from build123d import *

# Parameters (mm, degrees)
F1_DEPTH = 4
F2_R     = 5.08
F3_R     = 5.08
F4_R     = 1
F5_R     = 1
F6_R     = 1.5
F7_DEPTH = 25.4
F8_R     = 1


# Not quite as in the source:
# - a feature names something its author has since deleted; it is built from what else it names


with BuildPart() as f1:
    # F0 (on Top) → F1 (new body)
    with BuildSketch(Plane.XY):
        Polygon((0, -130), (0, 0), (-20.2767271549, 0), (-5.2268992042, -30.1366958052), align=None)
    extrude(amount=F1_DEPTH)

    # F2
    f2_edges = [f1.edges().sort_by_distance(p)[0] for p in [
        (0, 0, 2),
    ]]
    fillet(f2_edges, radius=F2_R)

    # F3
    f3_edges = [f1.edges().sort_by_distance(p)[0] for p in [
        (-20.276727, 0, 2),
    ]]
    fillet(f3_edges, radius=F3_R)

    # F4
    f4_edges = [f1.edges().sort_by_distance(p)[0] for p in [
        (0, -130, 2),
    ]]
    fillet(f4_edges, radius=F4_R)

    # F5
    f5_edges = [f1.edges().sort_by_distance(p)[0] for p in [
        (-10.916669, -18.743153, 4),
        (-3.612766, -60.975757, 4),
    ]]
    fillet(f5_edges, radius=F5_R)

    # F6 (on face) → F7 (cut)
    with BuildSketch(Plane.XY.offset(4)):
        with Locations((-13.589, -3.840335412)):
            Circle(F6_R)
        with Locations((-3.5482854582, -3.9438293315)):
            Circle(F6_R)
    extrude(amount=-F7_DEPTH, mode=Mode.SUBTRACT)

    # F8
    f8_edges = [f1.edges().sort_by_distance(p)[0] for p in [
        (-8.570816, 0, 0),
        (-10.916669, -18.743153, 0),
    ]]
    fillet(f8_edges, radius=F8_R)


solid = f1.part
The listing builds one solid part. Answer for the finished solid, in the listing's coordinates (mm). Give positions to 0.01 mm unless a question says otherwise; leave off trailing zeros. Order: outer loops, then holes, each group sorted by start corner. A loop starts at its lowest first (then second) coordinate and runs counter-clockwise, first axis right, second up. Notation, with made-up numbers: (59.5, 43) -> (111.5, 43) arc R25 cw to (111.5, 67) -> close; hole circle Ø8 at (-14, 44). An arc over 180 degrees is marked (long way). Put each result on its own line as item: value.
Item 1: Straight lines are drawn through the part: line 1 (Y direction, x = -14.75, z = 2.5); line 2 (Y direction, x = -12.5, z = 2.6); line 3 (X direction, y = -75.5, z = 3.35). For each, find the intervals that lie inside material, in ascending order.
Established:
line 1: y = -11.07 to -4.79, -2.89 to -0.77
line 2: y = -15.57 to -4.87, -2.81 to -0.02
line 3: x = -2.79 to -0.06
Item 2: Given P1, Ø1.5, axis at y = -55, z = 2.5, coming from the -X side; P2, Ø3.5, axis at x = -13.59, y = -3.84, coming from the -Z side; P3, Ø2, axis at y = -68.5, z = 1, coming from the -X side; P4, Ø6, axis at x = -5.5, y = -76.5, coming from the +Z side, each flat-ended and moving along its own axis, determine where each tip first touches the part or whether it passes through.
Established:
P1: stops at x = -3.96
P2: stops at z = 0
P3: stops at x = -3.27
P4: stops at z = 3.72
Item 3: For a pull along Y with two mould halves and no side action, classify faces 1 (the face through (-10.521, -18.863, 0.285)), 2 (the face through (-5.047, -3.878, 2.028)), 3 (the face through (-12.16, -3.39, 2.03)), 4 (the face through (0, -49, 2)) as released by +Y, released by -Y, zero draft, split by the parting line, or undercut.
Established:
face 1: released by -Y
face 2: undercut
face 3: undercut
face 4: zero draft
Item 4: A cutting plane is placed at A-A on z = 1.95. Give the vertices of the cut face in (x, y), plus the area to 3 significant figures.
Established:
outline: (-16.61, -7.35) -> (-5.23, -30.14) -> (-2, -91.81) arc R1 ccw to (0, -91.76) -> (0, -5.08) arc R5.08 ccw to (-5.08, 0) -> (-12.06, 0) arc R5.08 ccw to start; hole circle Ø3 at (-13.59, -3.84); hole circle Ø3 at (-3.55, -3.94)
area: 573 mm^2
